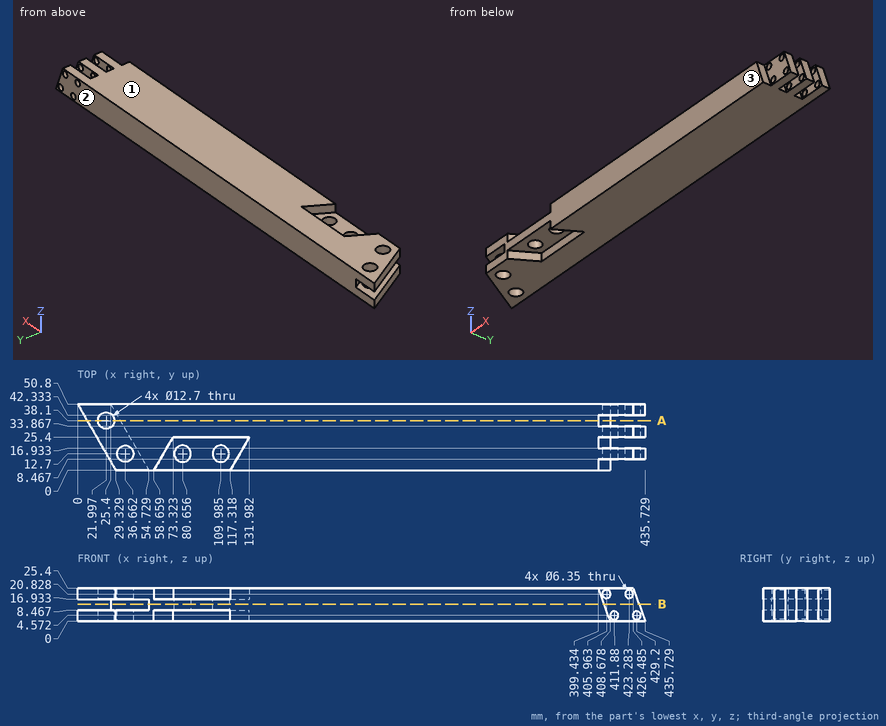
Study the drawing (mm; zero at the part's minimum x, y, z) and answer. Round coordinates to 2 decimals unless told otherwise and drop trailing zeros. Write each loop counter-clockwise with the first axis right and the second up, starting at its lowest first coordinate (ties: lowest second). Pieces come first, ordered by that corner, then holes. Notation, with made-up numbers: (10.5, 2) - (56.5, 2) arc R15 ccw to (56.5, 16) - close; hole circle Ø11 at (-33, 55.5). An arc over 180 degrees is marked (long way). Use a Markdown table: item, result. Add a question column.
1. The part is cut by section B-B (z = 13.25). Give the number of separate pieces and of enclosed holes in the cut face, and give its area (3 significant figures).
2. The part is cut by section A-A (y = 38.1). Write down the section's boundary in (x, z), and give its area (3 significant figures).
3. Flat-ended cylindrical pins translate along their axes: P1, Ø10, axis at x = 80.66, y = 12.7, coming from the -Z side; P2, Ø8.5, axis at x = 405.96, z = 20.83, coming from the -Y side; P3, Ø6, axis at y = 17.5, z = 5, coming from the -X side (1 decimal); P4, Ø3, axis at y = 30.5, z = 22.5, coming from the +X side (1 decimal). Find the tip coordinate at first contact, or state that the pin passes through.
4. Consider line 1 (X direction, y = 17, z = 6.25) (1 decimal); line 2 (X direction, y = 15.5, z = 1.75) (1 decimal); line 3 (X direction, y = 31, z = 21.25) (1 decimal). Determine where each line is inside the solid, lowest interval first.
5. For a pull along Y with two mould halves and no side action, classify the marked faces 1, 2 and 3 as +Y half, -Y half, draft (parallel to the pull), parting line (faces both ways), or undercut.
Reported:
| question | item | result |
|---|---|---|
| 1 | separate pieces | 1 |
| 1 | enclosed holes | 2 |
| 1 | area | 18,900 mm^2 |
| 2 | outline | (7.33, 0) - (15.65, 0) - (15.65, 8.47) - (7.33, 8.47) - close; (7.33, 16.93) - (15.65, 16.93) - (15.65, 25.4) - (7.33, 25.4) - close; (28.35, 0) - (408.68, 0) - (399.43, 25.4) - (28.35, 25.4) - (28.35, 16.93) - (32.73, 16.93) - (32.73, 8.47) - (28.35, 8.47) - close |
| 2 | area | 9,650 mm^2 |
| 3 | P1 | through |
| 3 | P2 | y = 8.47 |
| 3 | P3 | x = 17.5 |
| 3 | P4 | x = 428.1 |
| 4 | line 1 | 19.5 to 32, 41.3 to 68.5, 127.1 to 406.4 |
| 4 | line 2 | 20.4 to 31, 42.4 to 67.6, 126.3 to 410.4, 413.3 to 427.7, 430.7 to 435.1 |
| 4 | line 3 | 11.4 to 402.8, 409.1 to 420.1, 426.4 to 428 |
| 5 | face 1 | draft |
| 5 | face 2 | +Y half |
| 5 | face 3 | -Y half |
